Check sheet for the modelled part. Datum: model origin and axes. Units: mm. A direction names the side the tool comes from. Give positions to 0.01 mm unless a question says otherwise; leave off trailing zeros. Order: outer loops, then holes, each group sorted by start corner. A loop starts at its lowest first (then second) coordinate and runs counter-clockwise, first axis right, second up.
Item 1: Sectioned sample at C-C on z = 537.5. Record the boundary of the cut face in (x, y), and give its area (3 significant figures).
Item 2: Sectioned sample at A-A on x = 200. Record the boundary of the cut face in (y, z), and give its area (3 significant figures).
Item 3: Material ranges on line 1 along Y through (x, z) = (200, 444); line 2 along Z through (x, y) = (-259, -82); line 3 along X through (y, z) = (1, 261), recorded low to high.
Item 4: Gauge pin test, flat ends, axial feed: P1, Ø12, axis at x = -137.5, z = -41, coming from the +Y side; P2, Ø3, axis at y = -18.5, z = -41.5, coming from the -X side. Record the tip position at first contact, or that the pin passes through.
Item 5: Sectioned sample at B-B on y = 0. Record the boundary of the cut face in (x, z), and give its area (3 significant figures).
Item 6: Release check for a two-part mould opening along Y. For faces 3 (the cylindrical face through (-264.662, -26.81, -101.4)), 4 (the flat face through (-4, -100, 296)), 5 (the flat face through (-199, 1, -200)), 6 (the cylindrical face through (239.96, -1.76, 295.8)) record: released by +Y, released by -Y, zero draft, split by the parting line, or undercut.
Item 7: Access from +Z, -Z, +X, -X, +Y, -Y to the whole of each face (thin tool, end or side, straight path). Record for faces 1 (the cylindrical face through (-264.662, 26.81, 698.6)), 2 (the flat face through (300, -1, 296)).
Item 8: Sectioned sample at D-D on x = -200. Record the boundary of the cut face in (y, z).
from build123d import *

# Parameters (mm, degrees)
SKETCH1_W               = 600
SKETCH1_H               = 200
BOSS_EXTRUDE1_DEPTH     = 600
CUT_EXTRUDE1_DEPTH      = 40
CUT_EXTRUDE1_DEPTH_BACK = 600
SKETCH2_R               = 40
SKETCH3_R               = 70
BOSS_EXTRUDE2_DEPTH     = 200
BOSS_EXTRUDE3_START     = 200
SKETCH4_R               = 70
BOSS_EXTRUDE3_DEPTH     = 200


with BuildPart() as part:
    # Sketch1 → Boss-Extrude1 (new body)
    with BuildSketch(Plane.XY):
        Rectangle(SKETCH1_W, SKETCH1_H)
    extrude(amount=BOSS_EXTRUDE1_DEPTH)

    # Sketch2 → Cut-Extrude1 (cut, two sides: drawn at the far end of the back side and taken through both)
    with BuildSketch(Plane.XY.offset(600).offset(-CUT_EXTRUDE1_DEPTH_BACK)):
        with Locations(Location((200, 0, 0), (0, 0, 180))):
            Circle(SKETCH2_R)
    extrude(amount=CUT_EXTRUDE1_DEPTH + CUT_EXTRUDE1_DEPTH_BACK, mode=Mode.SUBTRACT)

    # Sketch3 → Boss-Extrude2 (add)
    with BuildSketch(Plane.XY.offset(600)):
        with Locations(Location((-200, 0, 0), (0, 0, 180))):
            Circle(SKETCH3_R)
    extrude(amount=BOSS_EXTRUDE2_DEPTH)

    # Sketch4 → Boss-Extrude3 (add)
    with BuildSketch(Plane(origin=(0, 0, 0), x_dir=(-1, 0, 0), z_dir=(0, 0, -1)).offset(BOSS_EXTRUDE3_START)):
        with Locations((200, 0)):
            Circle(SKETCH4_R)
    extrude(amount=-BOSS_EXTRUDE3_DEPTH)


solid = part.part
Report:
1. outline: (-300, -100) - (300, -100) - (300, 100) - (-300, 100) - close; hole circle Ø80 at (200, 0)
1. area: 115,000 mm2
2. outline: (-100, 0) - (-40, 0) - (-40, 600) - (-100, 600) - close; (40, 0) - (100, 0) - (100, 600) - (40, 600) - close
2. area: 72,000 mm2
3. line 1: y = -100 to -40, 40 to 100
3. line 2: z = 0 to 600
3. line 3: x = -300 to 160.01, 239.99 to 300
4. P1: stops at y = 41.32
4. P2: stops at x = -267.9
5. outline: (-300, 0) - (-270, 0) - (-270, -200) - (-130, -200) - (-130, 0) - (160, 0) - (160, 600) - (-130, 600) - (-130, 800) - (-270, 800) - (-270, 600) - (-300, 600) - close; (240, 0) - (300, 0) - (300, 600) - (240, 600) - close
5. area: 368,000 mm2
6. face 3: split by the parting line
6. face 4: released by -Y
6. face 5: zero draft
6. face 6: undercut
7. face 1: +Z
7. face 2: +Z, -Z, +X, +Y, -Y
8. outline: (-100, 0) - (-70, 0) - (-70, -200) - (70, -200) - (70, 0) - (100, 0) - (100, 600) - (70, 600) - (70, 800) - (-70, 800) - (-70, 600) - (-100, 600) - close
